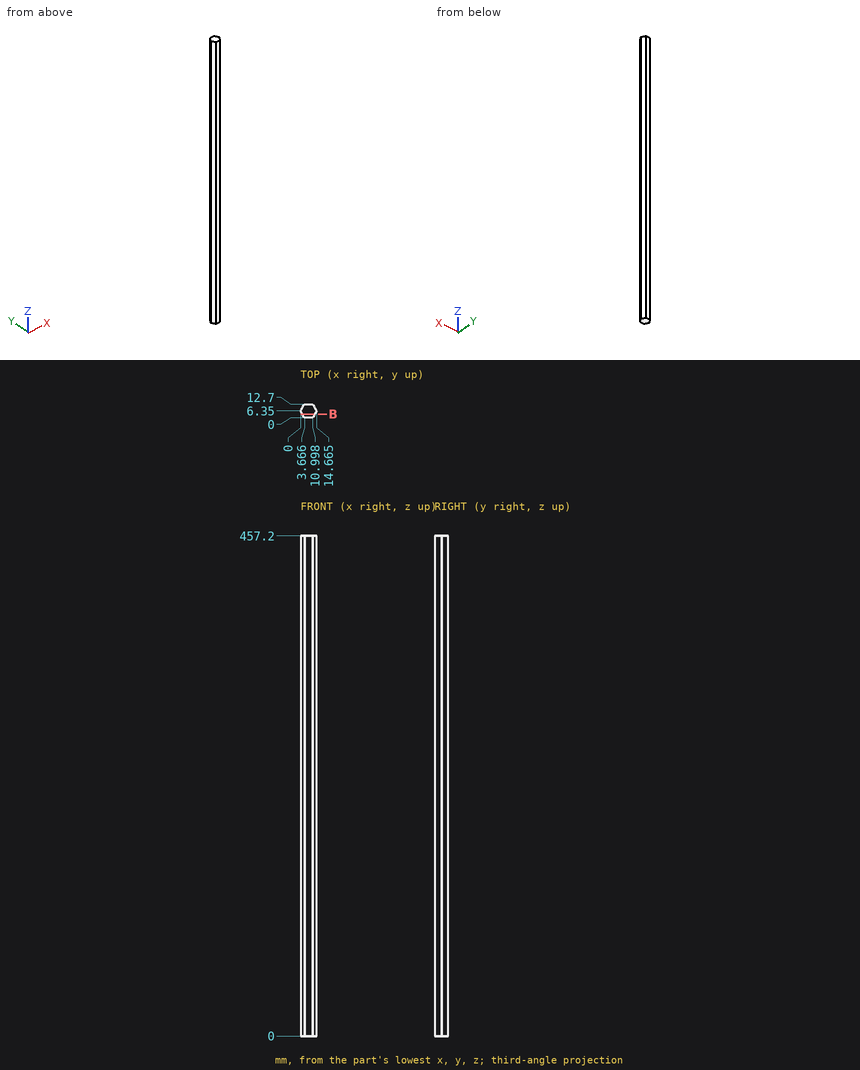
The drawing under review shows one solid part. Ordinate dimensions are in mm from its lowest x, y, z. Round coordinates to 2 decimals unless told otherwise and drop trailing zeros. Order: outer loops, then holes, each group sorted by start corner. A loop starts at its lowest first (then second) coordinate and runs counter-clockwise, first axis right, second up. Notation, with made-up numbers: (10, 89) -> (14, 89) arc R19 cw to (14, 100) -> close; hole circle Ø9 at (69.25, 45). An arc over 180 degrees is marked (long way). Use a Markdown table: item, result.
Item 1: For pin 1 (1.5 mm diameter, centred on y = 7.5, z = 348, fed in from +X) (1 decimal); pin 2 (2 mm diameter, centred on y = 11, z = 287, fed in from +X); pin 3 (4 mm diameter, centred on y = 2.5, z = 71.5, fed in from -X), all flat-tipped, find the tip position at first contact; note any pin that passes through.
Resolved:
| item | result |
|---|---|
| pin 1 | stops at x = 14.4 |
| pin 2 | stops at x = 12.56 |
| pin 3 | stops at x = 1.07 |
Item 2: Take a section at B-B (y = 3.5). State the section outline as (x, z) points (1 decimal), plus the area to 3 significant figures.
Resolved:
| item | result |
|---|---|
| outline | (1.6, 0) -> (13, 0) -> (13, 457.2) -> (1.6, 457.2) -> close |
| area | 5,200 mm² |
Item 3: For line 1 along Y through (x, z) = (11, 143) (1 decimal); line 2 along X through (y, z) = (5.25, 41) (1 decimal); line 3 along Y through (x, z) = (12, 287) (1 decimal), list the stretches that pass through material, from the lowest coordinate up. Write a range as [from, to].
Resolved:
| item | result |
|---|---|
| line 1 | y = [0, 12.7] |
| line 2 | x = [0.6, 14] |
| line 3 | y = [1.7, 11] |
